```python
from build123d import *

# Parameters (mm, degrees)
F0_W           = 20
F0_H           = 20
F1_DEPTH       = 25
F3_DEPTH       = 25
F4_R           = 2.5
F5_DEPTH       = 10
F7_R           = 5
F8_R           = 1
F10_DEPTH      = 20
F6_R           = 2.5
F11_DEPTH      = 15
F11_DEPTH_BACK = 25


with BuildPart() as f1:
    # F0 (on Top) → F1 (new body)
    with BuildSketch(Plane.XY):
        Rectangle(F0_W, F0_H)
    extrude(amount=F1_DEPTH)

    # F2 (on face) → F3 (cut)
    with BuildSketch(Plane(origin=(-10, 0, 0), x_dir=(0, -1, 0), z_dir=(-1, 0, 0))):
        Polygon((0, 15), (-10, 15), (-10, 8), (-4, 8), (-4, 6), (0, 6), (0, 8), align=None)
    extrude(amount=-F3_DEPTH, mode=Mode.SUBTRACT)

    # F4 (on face) → F5 (cut)
    with BuildSketch(Plane.XY.offset(25)):
        with Locations((0, 4.0342840366)):
            Circle(F4_R)
    extrude(amount=-F5_DEPTH, mode=Mode.SUBTRACT)

    # F7
    f7_edges = [f1.edges().sort_by_distance(p)[0] for p in [
        (0, 10, 0),
        (0, -10, 0),
    ]]
    fillet(f7_edges, radius=F7_R)

    # F8
    f8_edges = [f1.edges().sort_by_distance(p)[0] for p in [
        (0, 10, 15),
        (0, 10, 8),
        (0, 10, 25),
        (0, 4, 8),
    ]]
    fillet(f8_edges, radius=F8_R)

    # F9 (on face) → F10 (join)
    with BuildSketch(Plane(origin=(-10, 0, 0), x_dir=(0, -1, 0), z_dir=(-1, 0, 0))):
        Polygon((11.4480117336, 25), (10, 25), (10, 5), align=None)
    extrude(amount=-F10_DEPTH)

    # F6 (on face) → F11 (cut, two sides)
    with BuildSketch(Plane.XZ.offset(10)) as f11_sk:
        with Locations((-5.5, 20)):
            Circle(F6_R)
        with Locations((5.5, 20)):
            Circle(F6_R)
    extrude(amount=-F11_DEPTH, mode=Mode.SUBTRACT)
    extrude(f11_sk.sketch, amount=F11_DEPTH_BACK, mode=Mode.SUBTRACT)


solid = f1.part
```
Geometry check sheet. Reference: the model listing, model coordinates, mm. A direction names the side the tool comes from. Round coordinates to 2 decimals unless told otherwise and drop trailing zeros. Loops run counter-clockwise (first coordinate to the right, second up) from the corner with the lowest first, then second, coordinate; pieces in that order, holes last. Notation, with made-up numbers: M 75.25,-8.5 L 134.25,-8.5 A37 ccw 134.25,30.5 Z; hole C 71.25,36.25 d11. An arc over 180 degrees is marked long. Return JSON: item names as keys, results as strings. Group by question number.
(1) Section check A-A, the plane x = 0. Enter the section's corners in (y, z), and give its area (3 significant figures).
(2) Mould release check, pull along Y, two halves, no side actions. Record for faces 1 (the face through (5, 5, 20)), 2 (the face through (0, 7, 8)), 3 (the face through (0, 0, 10)): pulls with the +Y half, pulls with the -Y half, needs draft (parallel to the pull), parting line crosses it, or undercut.
(3) Go/stop test with flat-tipped pins: pin 1 (4 mm diameter, centred on x = -5.5, z = 21, fed in from -Y); pin 2 (1 mm diameter, centred on x = 7.5, z = 19.5, fed in from -Y); pin 3 (0.8 mm diameter, centred on x = 2.5, z = 6.5, fed in from -Y). Record where each tip stops, or that it passes through.
(4) Section check D-D, the plane y = -2.75. Enter the section's corners in (x, z).
(5) Scan lines: line 1 along X through (y, z) = (-7.25, 20); line 2 along Z through (x, y) = (5.5, 1.25); line 3 along Z through (x, y) = (-5.5, -1). Record each from-to range of solid material in increasing order. Write a range as [from, to].
(6) Set-up check for faces 4 (the face through (0.14, 9.715, 7.699)), 5 (the face through (-6, 5, 20)), 6 (the face through (-0.542, 1.594, 20.07)), 7 (the face through (-0.1, 4, 6.5)): record each of +Z, -Z, +X, -X, +Y, -Y from which the full face is reachable in a straight line by a thin tool's end or side.
(7) Section check B-B, the plane y = 2.25. Enter the section's corners in (x, z).
(8) Section check C-C, the plane z = 21.25. Enter the section's corners in (x, y).
Data:
{
 "1": {"outline": "M -11.45,25 L -10,5 A5 ccw -5,0 L 5,0 A5 ccw 10,5 L 10,7 A1 ccw 9,8 L 5,8 A1 ccw 4,7 L 4,6 L 0,6 L 0,15 L 1.53,15 L 1.53,25 Z; M 6.53,15 L 9,15 A1 ccw 10,16 L 10,24 A1 ccw 9,25 L 6.53,25 Z", "area": "375 mm²"},
 "2": {"face 1": "pulls with the -Y half", "face 2": "needs draft", "face 3": "undercut"},
 "3": {"pin 1": "y = -11.3", "pin 2": "y = -11.06", "pin 3": "y = -10.14"},
 "4": {"outline": "M -10,0 L 10,0 L 10,25 L -10,25 Z; hole C -5.5,20 d5; hole C 5.5,20 d5"},
 "5": {"line 1": "[-10, -8], [-3, 3], [8, 10]", "line 2": "[0, 6], [15, 17.5], [22.5, 25]", "line 3": "[0, 17.5], [22.5, 25]"},
 "6": {"face 4": "+X, -X, +Y", "face 5": "-Y", "face 6": "+Z", "face 7": "+X, -X"},
 "7": {"outline": "M -10,0 L 10,0 L 10,6 L -10,6 Z; M -10,15 L -1.75,15 L -1.75,25 L -10,25 Z; M 1.75,15 L 10,15 L 10,25 L 1.75,25 Z; hole C -5.5,20 d5; hole C 5.5,20 d5"},
 "8": {"outline": "M -10,-11.18 L -7.67,-11.18 L -7.67,5 L -3.33,5 L -3.33,-11.18 L 3.33,-11.18 L 3.33,5 L 7.67,5 L 7.67,-11.18 L 10,-11.18 L 10,10 L -10,10 Z; hole C 0,4.03 d5"}
}
